Autodesk Inventor part; units mm, degrees
ref_plane "YZ Plane" through (0, 0, 0) normal (1, 0, 0) x (0, 1, 0)
ref_plane "XZ Plane" through (0, 0, 0) normal (0, 1, 0) x (-1, 0, 0)
ref_plane "XY Plane" through (0, 0, 0) normal (0, 0, 1) x (1, 0, 0)
sketch "Эскиз1" plane through (0, 0, 0) normal (0, 1, 0) x (-1, 0, 0)
  line L0 (0, 0) -> (9, 0)
  line L1 (9, 0) -> (9, -35.56)
  line L2 (9, -35.56) -> (0, -35.56)
  line L3 (0, -35.56) -> (0, 0)
  line L4 (-8.5, -9.28) -> (7.5, -9.28)
  line L5 (8.5, -10.28) -> (8.5, -25.28)
  line L6 (7.5, -26.28) -> (-8.5, -26.28)
  line L7 (-8.5, -26.28) -> (-8.5, -9.28)
  line L8 (-8.5, -9.28) -> (8.5, -26.28) construction
  line L9 (8.5, -9.28) -> (-8.5, -26.28) construction
  circle A0 centre (7.5, -10.28) radius 1
  circle A1 centre (7.5, -25.28) radius 1
  line L10 (7.5, -9.28) -> (8.5, -9.28) construction
  line L11 (8.5, -10.28) -> (8.5, -9.28) construction
  line L12 (7.5, -26.28) -> (8.5, -26.28) construction
  line L13 (8.5, -26.28) -> (8.5, -25.28) construction
  line L14 (9, -25.28) -> (9, -10.28)
  line L15 (9, -10.28) -> (9, -8.78)
  line L16 (9, -8.78) -> (7.5, -8.78)
  line L17 (7.5, -8.78) -> (-9, -8.78)
  line L18 (-9, -8.78) -> (-9, -26.78)
  line L19 (-9, -26.78) -> (7.5, -26.78)
  line L20 (7.5, -26.78) -> (9, -26.78)
  line L21 (9, -26.78) -> (9, -25.28)
  line L22 (11, 2) -> (-2, 2)
  line L23 (-2, 2) -> (-2, -37.56)
  line L24 (-2, -37.56) -> (11, -37.56)
  line L25 (11, -37.56) -> (11, 2)
  line L26 (0, 2) -> (0, 0)
  line L27 (0, -35.56) -> (0, -37.56)
  circle A2 centre (5.7, -32.26) radius 1.6
  line L28 (0, -17.78) -> (11, -17.78) construction
  circle A3 centre (5.7, -3.3) radius 1.6
  point P0 (0, -26.78)
  point P1 (0, -8.78)
  dimension "d0" = 17
  dimension "d1" = 17
  dimension "d2" = 35.56
  dimension "d3" = 2
  dimension "d4" = 90
  dimension "d5" = 0.5
  dimension "d6" = 2
  dimension "d7" = 3.2
  dimension "d8" = 3.3
  dimension "d9" = 3.3
extrude "Выдавливание1" add sketch "Эскиз1" along normal blind 12 contours L26 L22 L25 L24 L27 L2 L1 L0 | L0 L1 L16 L17 L3 | L19 L20 L1 L2 L3
sketch "Эскиз2" plane through (0, 0, 0) normal (0, -1, 0) x (1, 0, 0)
  circle A0 centre (-5.7, -32.26) radius 1.6
  line L0 (-2.4668, -32.26) -> (-4.0834, -35.06)
  line L1 (-4.0834, -35.06) -> (-7.3166, -35.06)
  line L2 (-7.3166, -35.06) -> (-8.9332, -32.26)
  line L3 (-8.9332, -32.26) -> (-7.3166, -29.46)
  line L4 (-7.3166, -29.46) -> (-4.0834, -29.46)
  line L5 (-4.0834, -29.46) -> (-2.4668, -32.26)
  line L6 (-11, -37.56) -> (-11, 2)
  line L7 (-11, -17.78) -> (0, -17.78) construction
  circle A1 centre (-5.7, -3.3) radius 1.6
  line L8 (-2.4668, -3.3) -> (-4.0834, -0.5)
  line L9 (-4.0834, -0.5) -> (-7.3166, -0.5)
  line L10 (-7.3166, -0.5) -> (-8.9332, -3.3)
  line L11 (-8.9332, -3.3) -> (-7.3166, -6.1)
  line L12 (-7.3166, -6.1) -> (-4.0834, -6.1)
  line L13 (-4.0834, -6.1) -> (-2.4668, -3.3)
  point P0 (0, 0)
  dimension "d12" = 5.6
extrude "Выдавливание2" cut sketch "Эскиз2" against normal blind 2 contours L0 L1 L2 L3 L4 L5 | A1 | L13 L12 L11 L10 L9 L8
sketch "Эскиз3" plane through (0, 0, -26.78) normal (1, 0, 0) x (0, 0, -1)
  line L0 (-28.78, 0) -> (-28.78, 12)
  line L1 (10.78, 0) -> (-28.78, 0)
  line L2 (-28.78, 0) -> (-28.78, 12)
  line L3 (-28.78, 12) -> (10.78, 12)
  line L4 (10.78, 12) -> (10.78, 0)
  line L5 (8.78, 10) -> (-26.78, 10)
  line L6 (-26.78, 10) -> (-26.78, 2)
  line L7 (-26.78, 2) -> (8.78, 2)
  line L8 (8.78, 2) -> (8.78, 10)
  line L9 (10.78, 0) -> (10.78, 12)
  line L10 (-28.78, 0) -> (-18, 0)
  line L11 (8.78, 4) -> (-26.78, 4)
  point P0 (-26.78, 0)
  dimension "d15" = 2
  dimension "d16" = 2
extrude "Выдавливание3" cut sketch "Эскиз3" against normal up to surface (9 mm away) contours L8 L7 L6 L11
fillet "Сопряжение1" radius 1.3 4 edges at (-9, 1, -8.78) (-9, 8, -8.78) (-9, 1, -26.78) (-9, 8, -26.78)
sketch "Эскиз4" plane through (0, 12, 0) normal (0, 1, 0) x (1, 0, 0)
  line L0 (-7.7, 26.78) -> (0, 26.78)
  line L1 (-2.4, 26.78) -> (2.4, 26.78)
  line L2 (2.4, 26.78) -> (2.4, 28.28)
  line L3 (2.4, 28.28) -> (-2.4, 28.28)
  line L4 (-2.4, 28.28) -> (-2.4, 26.78)
  line L5 (0, 26.78) -> (-2.4, 28.28) construction
  line L6 (2.4, 28.28) -> (0, 26.78) construction
  line L7 (0, 26.78) -> (0, 37.56)
  circle A0 centre (0, 28.28) radius 2.4
  line L8 (0, 17.78) -> (-11, 17.78) construction
  line L9 (-11, 37.56) -> (-11, -2)
  line L10 (-2.4, 8.78) -> (2.4, 8.78)
  line L11 (2.4, 8.78) -> (2.4, 7.28)
  line L12 (2.4, 7.28) -> (-2.4, 7.28)
  line L13 (-2.4, 7.28) -> (-2.4, 8.78)
  line L14 (0, 8.78) -> (-2.4, 7.28) construction
  line L15 (2.4, 7.28) -> (0, 8.78) construction
  circle A1 centre (0, 7.28) radius 2.4
  line L16 (-11, -2) -> (0, 17.78) construction
  line L17 (0, 37.56) -> (-11, 37.56)
  line L18 (0, 17.78) -> (-11, 37.56) construction
  line L19 (-2.9, 26.28) -> (2.9, 26.28)
  line L20 (2.9, 26.28) -> (2.9, 28.78)
  line L21 (2.9, 28.78) -> (-2.9, 28.78)
  line L22 (-2.9, 28.78) -> (-2.9, 26.28)
  circle A2 centre (0, 28.28) radius 2.9
  circle A3 centre (0, 7.28) radius 2.9
  line L23 (2.9, 6.78) -> (2.9, 9.28)
  line L24 (2.9, 9.28) -> (-2.9, 9.28)
  line L25 (-2.9, 9.28) -> (-2.9, 6.78)
  line L26 (-2.9, 6.78) -> (2.9, 6.78)
  point P0 (0, 0)
  point P1 (-2.9, 28.28)
  point P2 (-2.9, 26.78)
  point P3 (0, 31.18)
  point P4 (1.8735, 8.78)
  point P5 (1.8735, 8.78)
  point P6 (-1.8735, 8.78)
  point P7 (-1.8735, 8.78)
  point P8 (-1.9, 8.7463)
  point P9 (-2.1, 9.28)
  point P10 (-2.9, 7.28)
  dimension "d20" = 4.8
  dimension "d21" = 1.5
  dimension "d22" = 0.5
  dimension "d23" = 0.5
extrude "Выдавливание4" cut sketch "Эскиз4" against normal up to surface (12 mm away) contours L22 A2 L0 | A2 L21 A0 L4 L0 | L4 A0 L0 | A2 L7 A0 L21 | A0 L3 L7 L0 | A0 L21 L7 L3 | A0 L7 L21 | L13 A1 L26 A3 L24 L10 | L10 A1 L13 | A1 L24 L10 | L10 A1 L12 | L12 A1 L26 | A1 L24 A3 L26 L11 L10 | L10 L11 A1 | L24 A3 A1 | A1 L24 | L26 A1 | A1 L26 A3 picked at (-0.403, 30.9667) picked at (-0.7824, 28.6133) picked at (-1.5074, 28.9517)
sketch "Эскиз5" plane through (0, 0, 2) normal (1, 0, 0) x (0, 0, -1)
  line L0 (10.78, 12) -> (10.78, 4)
  line L1 (2, 2) -> (2, 4)
  line L2 (2, 4) -> (10.78, 4)
  line L3 (10.78, 4) -> (10.78, 5.5)
  line L4 (10.78, 5.5) -> (2, 5.5)
  line L5 (2, 5.5) -> (2, 4)
  line L6 (30.28, 12) -> (30.28, 4)
  line L7 (37.56, 4) -> (37.56, 2)
  line L8 (33.18, 4) -> (37.56, 4)
  line L9 (37.56, 4) -> (30.28, 4)
  line L10 (30.28, 4) -> (30.28, 5.5)
  line L11 (30.28, 5.5) -> (37.56, 5.5)
  line L12 (37.56, 5.5) -> (37.56, 4)
  point P0 (2, 0)
  point P1 (10.78, 4)
  dimension "d26" = 1.5
extrude "Выдавливание5" cut sketch "Эскиз5" against normal blind 2
properties part number "krepl_1.2"
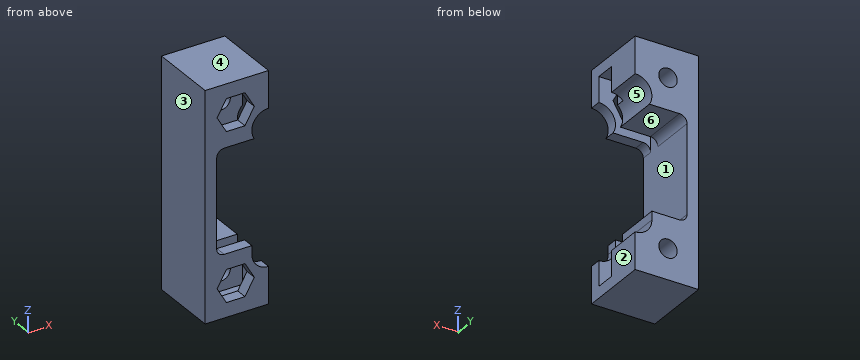
Verification items for the finished model (mm, model axes). Face numbers are marked on the shaded views. A direction names the side the tool comes from. Give positions to 0.01 mm unless a question says otherwise; leave off trailing zeros. Loops run counter-clockwise (first coordinate to the right, second up) from the corner with the lowest first, then second, coordinate; pieces in that order, holes last.
1) Sectioned sample at D-D, the plane y = 3. Enter the section's corners in (x, z), then the cut area to 3 significant figures.
2) Set-up check for the marked faces 1 and 2: record each of +Z, -Z, +X, -X, +Y, -Y from which the full face is reachable in a straight line by a thin tool's end or side.
3) Draft check along Z on the marked faces 3, 4, 5 and 6. Enter one of: pulls with the +Z half, pulls with the -Z half, needs draft (parallel to the pull), parting line crosses it, or undercut.
4) Depth check by flat-ended pin: pin 1 Ø1.6 at (x, z) = (-0.5, -31.5) entering from -Y; pin 2 Ø1.2 at (y, z) = (1.5, -28) entering from +X; pin 3 Ø2 at (x, z) = (-5, -31.5) entering from -Y. Enter the tip coordinate at first touch or a pass-through.
5) Sectioned sample at A-A, the plane x = -5.7. Count the separate pieces of the cut face and the enclosed holes in it, then the cut area to 3 significant figures.
6) Sectioned sample at C-C, the plane z = -2.5. Enter the section's corners in (x, y).
7) Thickness scan on line 1 along Z through (x, y) = (-5.7, 10); line 2 along Z through (x, y) = (-3.5, 9.5); line 3 along X through (y, z) = (6, -32.26). Record the ranges inside material, lowest first.
8) Sectioned sample at B-B, the plane y = 7. Enter the section's corners in (x, z).
Answers:
1. outline: (-11, -37.56) - (0, -37.56) - (0, -35.56) - (-9, -35.56) - (-9, 0) - (0, 0) - (0, 2) - (-11, 2) - close
1. area: 115 mm2
2. face 1: +X
2. face 2: +Z, -Z, +X, +Y, -Y
3. face 3: needs draft
3. face 4: pulls with the +Z half
3. face 5: undercut
3. face 6: undercut
4. pin 1: stops at y = 0
4. pin 2: stops at x = -2.88
4. pin 3: stops at y = 4
5. separate pieces: 6
5. enclosed holes: 0
5. area: 150 mm2
6. outline: (-11, 0) - (-8.47, 0) - (-8.47, 2) - (-9, 2) - (-9, 4) - (-7.09, 4) - (-7.09, 12) - (-11, 12) - close; (-4.31, 4) - (-2, 4) - (-2, 5.5) - (0, 5.5) - (0, 12) - (-4.31, 12) - close; (-2.93, 0) - (0, 0) - (0, 2) - (-2.93, 2) - close
7. line 1: z = -37.56 to -33.86, -30.66 to -26.78, -8.78 to -4.9, -1.7 to 2
7. line 2: z = -37.56 to -26.78, -8.78 to 2
7. line 3: x = -11 to -7.3, -4.1 to 0
8. outline: (-11, -37.56) - (0, -37.56) - (0, -31.18) arc R2.9 cw to (-2.9, -28.28) - (-2.9, -26.78) - (-7.7, -26.78) arc R1.3 cw to (-9, -25.48) - (-9, -10.08) arc R1.3 cw to (-7.7, -8.78) - (-2.48, -8.78) arc R2.9 cw to (0, -4.38) - (0, 2) - (-11, 2) - close; hole circle Ø3.2 at (-5.7, -32.26); hole circle Ø3.2 at (-5.7, -3.3)
